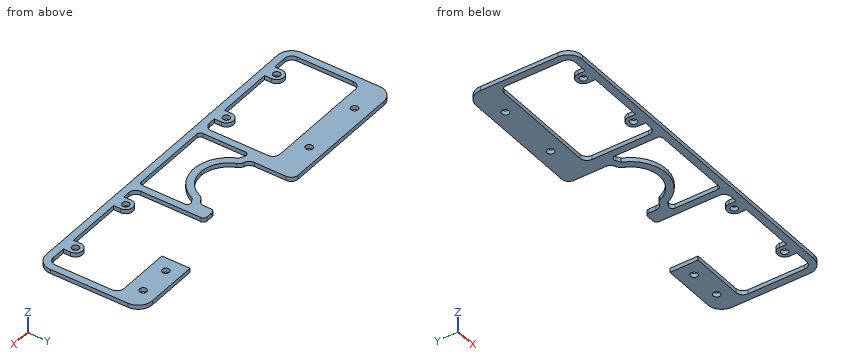
from build123d import *

# Parameters (mm, degrees)
BOSS_EXTRUDE1_DEPTH = 6
SKETCH3_R           = 5
CUT_EXTRUDE1_DEPTH  = 262.076617107
SKETCH4_R           = 5
CUT_EXTRUDE2_DEPTH  = 262.076617107
FILLET4_R           = 5
CUT_EXTRUDE5_DEPTH  = 262.076617107
FILLET5_R           = 5
FILLET6_R           = 5
CUT_EXTRUDE6_DEPTH  = 262.076617107
FILLET7_R           = 5


with BuildPart() as part:
    # Sketch1 → Boss-Extrude1 (new body)
    with BuildSketch(Plane.XY):
        with BuildLine():
            Line((-250, -55), (-250, 3.178280867))
            Line((-250, 3.178280867), (-250, 55))
            ThreePointArc((-250, 55), (-244.142135624, 69.142135624), (-230, 75))
            Line((-230, 75), (-220, 75))
            Line((-220, 75), (-164.330865428, 75))
            Line((-164.330865428, 75), (-60, 75))
            ThreePointArc((-60, 75), (-52.928932188, 72.071067812), (-50, 65))
            Line((-50, 65), (-50, 20))
            ThreePointArc((-50, 20), (-48.100925873, 14.1369803), (-43.125, 10.500822404))
            ThreePointArc((-43.125, 10.500822404), (-39.437786703, 8.32242004), (-37, 4.801315846))
            ThreePointArc((-37, 4.801315846), (-22.271648276, -13.226099426), (0, -20))
            Line((0, -20), (0, -40))
            Line((0, -40), (0, -65))
            Line((0, -65), (0, -75))
            Line((0, -75), (-230, -75))
            ThreePointArc((-230, -75), (-244.142135624, -69.142135624), (-250, -55))
        make_face()
    boss_extrude1 = extrude(amount=BOSS_EXTRUDE1_DEPTH)

    # Mirror1: Boss-Extrude1 across plane
    add(boss_extrude1.mirror(Plane(origin=(0, -20, 6), x_dir=(0, 0, 1), z_dir=(-1, 0, 0))))

    # Sketch3 → Cut-Extrude1 (cut, through all)
    with BuildSketch(Plane.XY.offset(6)):
        with BuildLine():
            Line((155, 35), (155, 75))
            Line((155, 75), (60, 75))
            ThreePointArc((60, 75), (52.928932188, 72.071067812), (50, 65))
            Line((50, 65), (50, 35))
            Line((50, 35), (155, 35))
        make_face()
        with Locations((175, 55)):
            Circle(SKETCH3_R)
        with Locations((220, 55)):
            Circle(SKETCH3_R)
        with Locations((-110, 55)):
            Circle(SKETCH3_R)
        with Locations((-200, 55)):
            Circle(SKETCH3_R)
    extrude(amount=-CUT_EXTRUDE1_DEPTH, mode=Mode.SUBTRACT)

    # Sketch4 → Cut-Extrude2 (cut, through all)
    with BuildSketch(Plane.XY.offset(6)):
        with Locations((-200, -55)):
            Circle(SKETCH4_R)
        with Locations((-100, -55)):
            Circle(SKETCH4_R)
        with BuildLine():
            Line((-70, 25.100979079), (-70, -54.899020921))
            ThreePointArc((-70, -54.899020921), (-72.928932188, -61.970088733), (-80, -64.899020921))
            Line((-80, -64.899020921), (-90, -64.899020921))
            Line((-90, -64.899020921), (-90, -55))
            ThreePointArc((-90, -55), (-100, -45), (-110, -55))
            Line((-110, -55), (-110, -65))
            Line((-110, -65), (-190, -65))
            Line((-190, -65), (-190, -55))
            ThreePointArc((-190, -55), (-200, -45), (-210, -55))
            Line((-210, -55), (-210, -65))
            Line((-210, -65), (-230, -65))
            ThreePointArc((-230, -65), (-237.071067812, -62.071067812), (-240, -55))
            Line((-240, -55), (-240, 25.100979079))
            ThreePointArc((-240, 25.100979079), (-237.071067812, 32.17204689), (-230, 35.100979079))
            Line((-230, 35.100979079), (-140, 35.100979079))
            Line((-140, 35.100979079), (-110, 35.100979079))
            Line((-110, 35.100979079), (-80, 35.100979079))
            ThreePointArc((-80, 35.100979079), (-72.928932188, 32.17204689), (-70, 25.100979079))
        make_face()
    cut_extrude2 = extrude(amount=-CUT_EXTRUDE2_DEPTH, mode=Mode.SUBTRACT)

    # Mirror2: Cut-Extrude2 across plane
    add(cut_extrude2.mirror(Plane(origin=(0, 0, 0), x_dir=(0, 0, 1), z_dir=(1, 0, 0))), mode=Mode.SUBTRACT)

    # Fillet4
    fillet4_edges = [part.edges().sort_by_distance(p)[0] for p in [
        (50, 35, 3),
    ]]
    fillet(fillet4_edges, radius=FILLET4_R)

    # Sketch8 → Cut-Extrude5 (cut, through all)
    with BuildSketch(Plane.XY.offset(6)):
        with BuildLine():
            Line((-60, 0), (-60, -64.899020921))
            Line((-60, -64.899020921), (60, -64.899020921))
            Line((60, -64.899020921), (60, 0))
            ThreePointArc((60, 0), (57.236067977, 4.472135955), (52, 4))
            ThreePointArc((52, 4), (49.247332505, 2.266223145), (46.25, 1.001644808))
            ThreePointArc((46.25, 1.001644808), (0, -30), (-46.25, 1.001644808))
            ThreePointArc((-46.25, 1.001644808), (-49.247332505, 2.266223145), (-52, 4))
            ThreePointArc((-52, 4), (-57.236067977, 4.472135955), (-60, 0))
        make_face()
    extrude(amount=-CUT_EXTRUDE5_DEPTH, mode=Mode.SUBTRACT)

    # Fillet5
    fillet5_edges = [part.edges().sort_by_distance(p)[0] for p in [
        (-60, -64.899020921, 3),
    ]]
    fillet(fillet5_edges, radius=FILLET5_R)

    # Fillet6
    fillet6_edges = [part.edges().sort_by_distance(p)[0] for p in [
        (60, -64.899020921, 3),
    ]]
    fillet(fillet6_edges, radius=FILLET6_R)

    # Sketch9 → Cut-Extrude6 (cut, through all)
    with BuildSketch(Plane.XY.offset(6)):
        with BuildLine():
            Line((78.582472294, 35), (70, 35))
            Line((70, 35), (70, 25.100979079))
            ThreePointArc((70, 25.100979079), (72.444363791, 31.651731819), (78.582472294, 35))
        make_face()
    extrude(amount=-CUT_EXTRUDE6_DEPTH, mode=Mode.SUBTRACT)

    # Fillet7
    fillet7_edges = [part.edges().sort_by_distance(p)[0] for p in [
        (70, 35, 3),
    ]]
    fillet(fillet7_edges, radius=FILLET7_R)


solid = part.part
Can you work these out from the model? Positions are in its coordinate system, mm. Round coordinates to 2 decimals unless told otherwise and drop trailing zeros. Loops run counter-clockwise (first coordinate to the right, second up) from the corner with the lowest first, then second, coordinate; pieces in that order, holes last. Notation, with made-up numbers: (83, 31.5) - (141, 31.5) arc R6 cw to (141, 40.5) - close; hole circle Ø7 at (20.5, -15.75). An arc over 180 degrees is marked (long way). Write item = value, one per line. Start each with the question number.
(1) If we section it at C-C (x = -200): Please give me the cut outline in (y, z).
(2) If we section it at B-B (x = 100): Please give me the cut outline in (y, z).
(3) For P1, Ø3, axis at x = 57.5, z = 3.5, coming from the +Y side; P2, Ø3, axis at y = -59.5, z = 4, coming from the +X side, each with a flat end and sliding along its axis, tell me the tip position at first contact or that it passes through.
(4) If I drill on probe 1 along Y at (x, z) = (-100, 2.9); probe 2 along Y at (x, z) = (-200, 4.35); probe 3 along Y at (x, z) = (-116.5, 5.35), over which ranges is the centre line in solid material (lowest first)? Write a range as [from, to].
(5) If we section it at D-D (z = 3.35): Give the number of separate pieces and of enclosed holes in the cut face, and give its area (3 significant figures).
(6) If we section it at A-A (x = 200): Please give me the cut outline in (y, z), and give its area (3 significant figures).
Ans:
q1.outline = (-75, 0) - (-60, 0) - (-60, 6) - (-75, 6) - close; (-50, 0) - (-45, 0) - (-45, 6) - (-50, 6) - close; (35.1, 0) - (50, 0) - (50, 6) - (35.1, 6) - close; (60, 0) - (75, 0) - (75, 6) - (60, 6) - close
q2.outline = (-75, 0) - (-60, 0) - (-60, 6) - (-75, 6) - close; (-50, 0) - (-45, 0) - (-45, 6) - (-50, 6) - close
q3.P1 = 35
q3.P2 = 249.77
q4.probe_1 = [-75, -60], [-50, -45], [35.1, 75]
q4.probe_2 = [-75, -60], [-50, -45], [35.1, 50], [60, 75]
q4.probe_3 = [-75, -65], [35.1, 75]
q5.separate_pieces = 1
q5.enclosed_holes = 10
q5.area = 23,300 mm²
q6.outline = (-75, 0) - (-60, 0) - (-60, 6) - (-75, 6) - close; (-50, 0) - (-45, 0) - (-45, 6) - (-50, 6) - close; (35.1, 0) - (75, 0) - (75, 6) - (35.1, 6) - close
q6.area = 359 mm²
